```python
from build123d import *

# Parameters (mm, degrees)
BOSS_EXTRUDE1_DEPTH     = 139
SKETCH3_R               = 2
CUT_EXTRUDE1_DEPTH      = 153.647469681
SKETCH5_W               = 30
SKETCH5_H               = 60
BOSS_EXTRUDE2_DEPTH     = 13.7
SKETCH6_W               = 27.582278357
SKETCH6_H               = 4.25
SKETCH6_W_2             = 27.382278357
BOSS_EXTRUDE3_DEPTH     = 10
CUT_EXTRUDE3_DEPTH      = 132.062650228
CUT_EXTRUDE3_DEPTH_BACK = 132.062650228
SKETCH7_R               = 1
SKETCH4_R               = 7.5
BOSS_EXTRUDE4_DEPTH     = 52
BOSS_EXTRUDE5_START     = -155
SKETCH4_2_R             = 7.5
BOSS_EXTRUDE5_DEPTH     = 155
SKETCH8_W               = 30
SKETCH8_H               = 13.7
CUT_EXTRUDE4_DEPTH      = 18.85
SKETCH9_W               = 95.207004137
SKETCH9_H               = 27
CUT_EXTRUDE5_DEPTH      = 202.60032242
SKETCH10_W              = 139
SKETCH10_H              = 30
CUT_EXTRUDE6_DEPTH      = 16.5
CUT_EXTRUDE7_DEPTH      = 203.936541806
CUT_EXTRUDE7_DEPTH_BACK = 13.7
SKETCH11_W              = 30
SKETCH11_H              = 45.211643816
SKETCH12_W              = 139
SKETCH12_H              = 13
CUT_EXTRUDE8_DEPTH      = 202.149819786
CUT_EXTRUDE9_REACH      = 199.662
SKETCH13_R              = 2.5
SKETCH14_W              = 22
SKETCH14_H              = 27
CUT_EXTRUDE10_DEPTH     = 8


with BuildPart() as part:
    # Sketch2 → Boss-Extrude1 (new body)
    with BuildSketch(Plane(origin=(0, 0, 0), x_dir=(0, 0, -1), z_dir=(1, 0, 0))):
        Polygon((-6.75, 30), (6.75, 30), (6.75, 60), (9.75, 60), (9.75, 51.134717436), (9.75, 0), (-9.75, 0), (-9.75, 60), (-6.75, 60), align=None)
    extrude(amount=BOSS_EXTRUDE1_DEPTH)

    # Sketch3 → Cut-Extrude1 (cut, through all)
    with BuildSketch(Plane(origin=(0, 0, -9.75), x_dir=(-1, 0, 0), z_dir=(0, 0, -1))):
        with Locations((-119, 40)):
            Circle(SKETCH3_R)
        with BuildLine():
            Line((-85, 42), (-15, 42))
            ThreePointArc((-15, 42), (-13, 40), (-15, 38))
            Line((-15, 38), (-85, 38))
            ThreePointArc((-85, 38), (-87, 40), (-85, 42))
        make_face()
    extrude(amount=-CUT_EXTRUDE1_DEPTH, mode=Mode.SUBTRACT)

    # Sketch5 → Boss-Extrude2 (add)
    with BuildSketch(Plane(origin=(0, 0, -9.75), x_dir=(-1, 0, 0), z_dir=(0, 0, -1))):
        with Locations((-124, 30)):
            Rectangle(SKETCH5_W, SKETCH5_H)
    extrude(amount=BOSS_EXTRUDE2_DEPTH)

    # Sketch6 → Boss-Extrude3 (add)
    with BuildSketch(Plane(origin=(0, 0, -23.45), x_dir=(-1, 0, 0), z_dir=(0, 0, -1))):
        with Locations((-125.208860821, 20.975)):
            Rectangle(SKETCH6_W, SKETCH6_H)
        with Locations((-125.308860822, 48.775)):
            Rectangle(SKETCH6_W_2, SKETCH6_H)
    extrude(amount=BOSS_EXTRUDE3_DEPTH)

    # Sketch7 → Cut-Extrude3 (cut, two sides: drawn at the far end of the back side and taken through both)
    with BuildSketch(Plane.ZY.offset(-111.617721643).offset(-CUT_EXTRUDE3_DEPTH_BACK)):
        with Locations((-30.95, 48.78)):
            Circle(SKETCH7_R)
        with Locations((-30.95, 20.97)):
            Circle(SKETCH7_R)
    extrude(amount=CUT_EXTRUDE3_DEPTH + CUT_EXTRUDE3_DEPTH_BACK, mode=Mode.SUBTRACT)

    # Sketch4 → Boss-Extrude4 (add)
    with BuildSketch(Plane(origin=(139, 0, 0), x_dir=(0, 0, -1), z_dir=(1, 0, 0))):
        with Locations(Location((-2.25, 15, 0), (0, 0, 180))):
            Circle(SKETCH4_R)
    extrude(amount=BOSS_EXTRUDE4_DEPTH)

    # Sketch4<2> → Boss-Extrude5 (add)
    with BuildSketch(Plane(origin=(139, 0, 0), x_dir=(0, 0, -1), z_dir=(1, 0, 0)).offset(BOSS_EXTRUDE5_START)):
        with Locations(Location((-2.25, 15, 0), (0, 0, 180))):
            Circle(SKETCH4_2_R)
    extrude(amount=BOSS_EXTRUDE5_DEPTH)

    # Sketch8 → Cut-Extrude4 (cut)
    with BuildSketch(Plane.XZ):
        with Locations((124, -16.6)):
            Rectangle(SKETCH8_W, SKETCH8_H)
    extrude(amount=-CUT_EXTRUDE4_DEPTH, mode=Mode.SUBTRACT)

    # Sketch9 → Cut-Extrude5 (cut, through all)
    with BuildSketch(Plane(origin=(0, 0, -9.75), x_dir=(-1, 0, 0), z_dir=(0, 0, -1))):
        with Locations((-61.396497932, 13.5)):
            Rectangle(SKETCH9_W, SKETCH9_H)
    extrude(amount=-CUT_EXTRUDE5_DEPTH, mode=Mode.SUBTRACT)

    # Sketch10 → Cut-Extrude6 (cut)
    with BuildSketch(Plane.XY.offset(9.75)):
        with Locations((69.5, 45)):
            Rectangle(SKETCH10_W, SKETCH10_H)
    extrude(amount=-CUT_EXTRUDE6_DEPTH, mode=Mode.SUBTRACT)

    # Sketch11 → Cut-Extrude7 (cut, two sides: drawn at the far end of the back side and taken through both)
    with BuildSketch(Plane(origin=(0, 0, -23.45), x_dir=(-1, 0, 0), z_dir=(0, 0, -1)).offset(-CUT_EXTRUDE7_DEPTH_BACK)):
        with Locations((-124, 37.394178092)):
            Rectangle(SKETCH11_W, SKETCH11_H)
    extrude(amount=CUT_EXTRUDE7_DEPTH + CUT_EXTRUDE7_DEPTH_BACK, mode=Mode.SUBTRACT)

    # Sketch12 → Cut-Extrude8 (cut, through all)
    with BuildSketch(Plane(origin=(0, 0, -9.75), x_dir=(-1, 0, 0), z_dir=(0, 0, -1))):
        with Locations((-69.5, 53.5)):
            Rectangle(SKETCH12_W, SKETCH12_H)
    extrude(amount=-CUT_EXTRUDE8_DEPTH, mode=Mode.SUBTRACT)

    # Sketch13 → Cut-Extrude9 (cut, up to next)
    with BuildSketch(Plane(origin=(0, 0, -9.75), x_dir=(-1, 0, 0), z_dir=(0, 0, -1)), mode=Mode.PRIVATE) as cut_extrude9_sk1:
        with Locations((-126, 7)):
            Circle(SKETCH13_R)
    cut_extrude9_tool1 = extrude(cut_extrude9_sk1.sketch, amount=-CUT_EXTRUDE9_REACH, mode=Mode.PRIVATE) & part.part
    # Sketch13 → Cut-Extrude9 (cut, up to next)
    with BuildSketch(Plane(origin=(0, 0, -9.75), x_dir=(-1, 0, 0), z_dir=(0, 0, -1)), mode=Mode.PRIVATE) as cut_extrude9_sk2:
        with Locations((-126, 17)):
            Circle(SKETCH13_R)
    cut_extrude9_tool2 = extrude(cut_extrude9_sk2.sketch, amount=-CUT_EXTRUDE9_REACH, mode=Mode.PRIVATE) & part.part
    add(cut_extrude9_tool1.solids().sort_by_distance((126, 7, -9.75))[0], mode=Mode.SUBTRACT)
    add(cut_extrude9_tool2.solids().sort_by_distance((126, 17, -9.75))[0], mode=Mode.SUBTRACT)

    # Sketch14 → Cut-Extrude10 (cut)
    with BuildSketch(Plane.XY.offset(9.75)):
        with Locations((120, 13.5)):
            Rectangle(SKETCH14_W, SKETCH14_H)
    extrude(amount=-CUT_EXTRUDE10_DEPTH, mode=Mode.SUBTRACT)


solid = part.part
```
Build history of the part. All positions in model axes, mm. A direction names the side the tool comes from. Coordinates: 2 decimals unless noted, no trailing zeros. Order: outer loops, then holes, each group sorted by start corner. A loop starts at its lowest first (then second) coordinate and runs counter-clockwise, first axis right, second up.
Item 1: Tool access for faces 4 (the flat face through (69, 30, 2)), 5 (the flat face through (13.793, 13, 0)), 6 (the cylindrical face through (-8.11, 22.32, 0.62)), 7 (the flat face through (131, 13, 6)): list every direction of +Z, -Z, +X, -X, +Y, -Y with a clear straight run to the whole face (end or side of a thin tool).
Filled in:
face 4: +Z, +X, -X, +Y
face 5: +Z, -Z, -Y
face 6: -X
face 7: +Z, -Y
Item 2: Saw through at D-D on x = 97. List the corners of the cut face in (y, z).
Filled in:
outline: (27, -9.75) - (47, -9.75) - (47, -6.75) - (30, -6.75) - (30, 9.75) - (27, 9.75) - close
Item 3: Saw through at C-C on x = 20.5. List the corners of the cut face in (y, z), then the cut area to 3 significant figures.
Filled in:
outline: (27, -9.75) - (38, -9.75) - (38, -6.75) - (30, -6.75) - (30, 9.75) - (27, 9.75) - close; (42, -9.75) - (47, -9.75) - (47, -6.75) - (42, -6.75) - close
area: 97.5 mm2
Item 4: Drill centre lines: L1, parallel to Y at x = 126, z = -5; L2, parallel to Y at x = 119, z = -7.4; L3, parallel to X at y = 26.5, z = 2.75. Where is each one in solid material? Low to high.
Filled in:
L1: y = 0 to 4.5, 9.5 to 14.5, 19.5 to 30
L2: y = 0 to 38, 42 to 47
L3: x = 0 to 13.79, 131 to 139
Item 5: Mould opens along Y. For faces 1 (the cylindrical face through (164.64, 22.32, 0.62)), 2 (the flat face through (120, 14, 1.75)), 3 (the cylindrical face through (123.615, 17.751, -4.08)) say: released by +Y, released by -Y, zero draft, split by the parting line, or undercut.
Filled in:
face 1: split by the parting line
face 2: zero draft
face 3: undercut
Item 6: Saw through at B-B on y = 17. List the corners of the cut face in (x, z).
Filled in:
outline: (-16, -4.98) - (0, -4.98) - (0, -9.75) - (13.79, -9.75) - (13.79, 9.75) - (0, 9.75) - (0, 9.48) - (-16, 9.48) - close; (109, -9.75) - (123.5, -9.75) - (123.5, 1.75) - (109, 1.75) - close; (128.5, -9.75) - (139, -9.75) - (139, -4.98) - (191, -4.98) - (191, 9.48) - (139, 9.48) - (139, 9.75) - (131, 9.75) - (131, 1.75) - (128.5, 1.75) - close
Item 7: Saw through at A-A on x = 119. List the corners of the cut face in (y, z).
Filled in:
outline: (0, -9.75) - (38, -9.75) - (38, -6.75) - (30, -6.75) - (30, 9.75) - (27, 9.75) - (27, 1.75) - (0, 1.75) - close; (42, -9.75) - (47, -9.75) - (47, -6.75) - (42, -6.75) - close
Item 8: Drop flat-ended pins along their axis: pin 1 Ø5 at (y, z) = (28, -6) entering from -X; pin 2 Ø1.5 at (y, z) = (28, -3.5) entering from +X; pin 3 Ø1.5 at (x, z) = (48, -8.5) entering from -Y. Give the stop position or say it passes through.
Filled in:
pin 1: stops at x = 0
pin 2: stops at x = 139
pin 3: stops at y = 27
